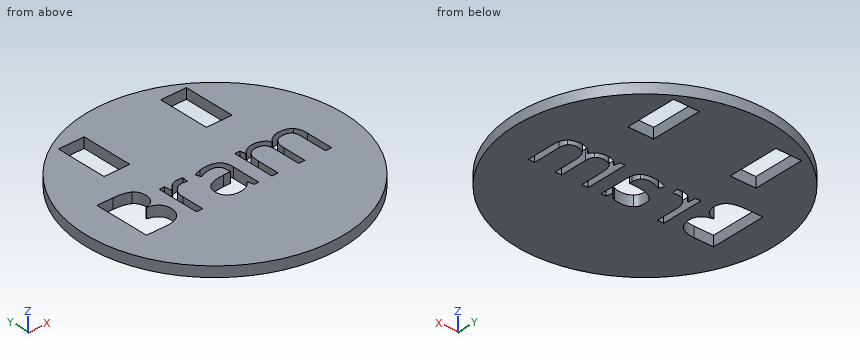
from build123d import *

# Parameters (mm, degrees)
F0_R     = 25
F0_W     = 5
F0_H     = 10
F1_DEPTH = 2


with BuildPart() as f1:
    # F0 (on Top) → F1 (new body)
    with BuildSketch(Plane.XY):
        Circle(F0_R)
        with BuildLine():
            Line((-18.475540486, -5.8509828523), (-18.475540486, 5.0045425299))
            Line((-18.475540486, 5.0045425299), (-15.4082427691, 5.0045425299))
            add(Edge.make_bspline(
                [(-15.4082427691, 5.0045425299), (-13.2485420529, 5.0045425299), (-12.2827352969, 4.3582954509)],
                knots=[0, 0, 0, 1, 1, 1], degree=2))
            add(Edge.make_bspline(
                [(-12.2827352969, 4.3582954509), (-11.316928541, 3.7120483719), (-11.316928541, 2.3173901536)],
                knots=[0, 0, 0, 1, 1, 1], degree=2))
            add(Edge.make_bspline(
                [(-11.316928541, 2.3173901536), (-11.316928541, 1.3503954435), (-11.8550717888, 0.7231556315)],
                knots=[0, 0, 0, 1, 1, 1], degree=2))
            add(Edge.make_bspline(
                [(-11.8550717888, 0.7231556315), (-12.3932150366, 0.0959158196), (-13.4267351813, -0.089405034)],
                knots=[0, 0, 0, 1, 1, 1], degree=2))
            Line((-13.4267351813, -0.089405034), (-13.4267351813, -0.1630581937))
            add(Edge.make_bspline(
                [(-13.4267351813, -0.1630581937), (-10.9534145591, -0.5859698851), (-10.9534145591, -2.76230196)],
                knots=[0, 0, 0, 1, 1, 1], degree=2))
            add(Edge.make_bspline(
                [(-10.9534145591, -2.76230196), (-10.9534145591, -4.2163578877), (-11.9370406278, -5.03367037)],
                knots=[0, 0, 0, 1, 1, 1], degree=2))
            add(Edge.make_bspline(
                [(-11.9370406278, -5.03367037), (-12.9206666966, -5.8509828523), (-14.6883425304, -5.8509828523)],
                knots=[0, 0, 0, 1, 1, 1], degree=2))
            Line((-14.6883425304, -5.8509828523), (-18.475540486, -5.8509828523))
        make_face(mode=Mode.SUBTRACT)
        with BuildLine():
            add(Edge.make_bspline(
                [(-6.4985863491, 2.0049582018), (-5.8594669952, 2.4361855726), (-5.0944244973, 2.4361855726)],
                knots=[0, 0, 0, 1, 1, 1], degree=2))
            add(Edge.make_bspline(
                [(-5.0944244973, 2.4361855726), (-4.5527173869, 2.4361855726), (-4.1226779704, 2.3459010542)],
                knots=[0, 0, 0, 1, 1, 1], degree=2))
            Line((-4.1226779704, 2.3459010542), (-4.2937433736, 1.203089124))
            add(Edge.make_bspline(
                [(-4.2937433736, 1.203089124), (-4.7974359499, 1.3147568178), (-5.1847090156, 1.3147568178)],
                knots=[0, 0, 0, 1, 1, 1], degree=2))
            add(Edge.make_bspline(
                [(-5.1847090156, 1.3147568178), (-6.1730869012, 1.3147568178), (-6.8739798729, 0.51288774)],
                knots=[0, 0, 0, 1, 1, 1], degree=2))
            add(Edge.make_bspline(
                [(-6.8739798729, 0.51288774), (-7.5748728446, -0.2889813378), (-7.5748728446, -1.4840632523)],
                knots=[0, 0, 0, 1, 1, 1], degree=2))
            Line((-7.5748728446, -1.4840632523), (-7.5748728446, -5.8509828523))
            Line((-7.5748728446, -5.8509828523), (-8.8079692931, -5.8509828523))
            Line((-8.8079692931, -5.8509828523), (-8.8079692931, 2.2865033447))
            Line((-8.8079692931, 2.2865033447), (-7.7910805071, 2.2865033447))
            Line((-7.7910805071, 2.2865033447), (-7.6485260043, 0.7801774326))
            Line((-7.6485260043, 0.7801774326), (-7.5891282949, 0.7801774326))
            add(Edge.make_bspline(
                [(-7.5891282949, 0.7801774326), (-7.1377057029, 1.5737308311), (-6.4985863491, 2.0049582018)],
                knots=[0, 0, 0, 1, 1, 1], degree=2))
        make_face(mode=Mode.SUBTRACT)
        with BuildLine():
            Line((3.3186670717, -5.8509828523), (2.4039423459, -5.8509828523))
            Line((2.4039423459, -5.8509828523), (2.1592237829, -4.6915395635))
            Line((2.1592237829, -4.6915395635), (2.0998260734, -4.6915395635))
            add(Edge.make_bspline(
                [(2.0998260734, -4.6915395635), (1.4915935284, -5.4565820614), (0.8869248461, -5.7286235708)],
                knots=[0, 0, 0, 1, 1, 1], degree=2))
            add(Edge.make_bspline(
                [(0.8869248461, -5.7286235708), (0.2822561637, -6.0006650801), (-0.625340837, -6.0006650801)],
                knots=[0, 0, 0, 1, 1, 1], degree=2))
            add(Edge.make_bspline(
                [(-0.625340837, -6.0006650801), (-1.8346782017, -6.0006650801), (-2.5213157231, -5.3758011765)],
                knots=[0, 0, 0, 1, 1, 1], degree=2))
            add(Edge.make_bspline(
                [(-2.5213157231, -5.3758011765), (-3.2079532446, -4.750937273), (-3.2079532446, -3.6009976177)],
                knots=[0, 0, 0, 1, 1, 1], degree=2))
            add(Edge.make_bspline(
                [(-3.2079532446, -3.6009976177), (-3.2079532446, -1.137180629), (0.7336787556, -1.01838521)],
                knots=[0, 0, 0, 1, 1, 1], degree=2))
            Line((0.7336787556, -1.01838521), (2.1140815237, -0.9732429509))
            Line((2.1140815237, -0.9732429509), (2.1140815237, -0.4671744662))
            add(Edge.make_bspline(
                [(2.1140815237, -0.4671744662), (2.1140815237, 0.4903166104), (1.7030493742, 0.9464910191)],
                knots=[0, 0, 0, 1, 1, 1], degree=2))
            add(Edge.make_bspline(
                [(1.7030493742, 0.9464910191), (1.2920172246, 1.4026654278), (0.384420224, 1.4026654278)],
                knots=[0, 0, 0, 1, 1, 1], degree=2))
            add(Edge.make_bspline(
                [(0.384420224, 1.4026654278), (-0.6324685621, 1.4026654278), (-1.9154590866, 0.7801774326)],
                knots=[0, 0, 0, 1, 1, 1], degree=2))
            Line((-1.9154590866, 0.7801774326), (-2.2956044272, 1.723413059))
            add(Edge.make_bspline(
                [(-2.2956044272, 1.723413059), (-1.6944996074, 2.0489125068), (-0.9781632312, 2.2342333604)],
                knots=[0, 0, 0, 1, 1, 1], degree=2))
            add(Edge.make_bspline(
                [(-0.9781632312, 2.2342333604), (-0.261826855, 2.4195542139), (0.4604492921, 2.4195542139)],
                knots=[0, 0, 0, 1, 1, 1], degree=2))
            add(Edge.make_bspline(
                [(0.4604492921, 2.4195542139), (1.9145052199, 2.4195542139), (2.6165861458, 1.7744950891)],
                knots=[0, 0, 0, 1, 1, 1], degree=2))
            add(Edge.make_bspline(
                [(2.6165861458, 1.7744950891), (3.3186670717, 1.1294359643), (3.3186670717, -0.2961090629)],
                knots=[0, 0, 0, 1, 1, 1], degree=2))
            Line((3.3186670717, -0.2961090629), (3.3186670717, -5.8509828523))
        make_face(mode=Mode.SUBTRACT)
        with BuildLine():
            Line((17.4600737416, -5.8509828523), (16.2293532014, -5.8509828523))
            Line((16.2293532014, -5.8509828523), (16.2293532014, -0.5574589846))
            add(Edge.make_bspline(
                [(16.2293532014, -0.5574589846), (16.2293532014, 0.4166634507), (15.8135692351, 0.9025367141)],
                knots=[0, 0, 0, 1, 1, 1], degree=2))
            add(Edge.make_bspline(
                [(15.8135692351, 0.9025367141), (15.3977852689, 1.3884099776), (14.5210750771, 1.3884099776)],
                knots=[0, 0, 0, 1, 1, 1], degree=2))
            add(Edge.make_bspline(
                [(14.5210750771, 1.3884099776), (13.3711354218, 1.3884099776), (12.8211126322, 0.7279074483)],
                knots=[0, 0, 0, 1, 1, 1], degree=2))
            add(Edge.make_bspline(
                [(12.8211126322, 0.7279074483), (12.2710898425, 0.067404919), (12.2710898425, -1.3058701239)],
                knots=[0, 0, 0, 1, 1, 1], degree=2))
            Line((12.2710898425, -1.3058701239), (12.2710898425, -5.8509828523))
            Line((12.2710898425, -5.8509828523), (11.037993394, -5.8509828523))
            Line((11.037993394, -5.8509828523), (11.037993394, -0.5574589846))
            add(Edge.make_bspline(
                [(11.037993394, -0.5574589846), (11.037993394, 0.4166634507), (10.6222094277, 0.9025367141)],
                knots=[0, 0, 0, 1, 1, 1], degree=2))
            add(Edge.make_bspline(
                [(10.6222094277, 0.9025367141), (10.2064254614, 1.3884099776), (9.3225875446, 1.3884099776)],
                knots=[0, 0, 0, 1, 1, 1], degree=2))
            add(Edge.make_bspline(
                [(9.3225875446, 1.3884099776), (8.1655201642, 1.3884099776), (7.6273769164, 0.694644731)],
                knots=[0, 0, 0, 1, 1, 1], degree=2))
            add(Edge.make_bspline(
                [(7.6273769164, 0.694644731), (7.0892336686, 0.0008794844), (7.0892336686, -1.5814754958)],
                knots=[0, 0, 0, 1, 1, 1], degree=2))
            Line((7.0892336686, -1.5814754958), (7.0892336686, -5.8509828523))
            Line((7.0892336686, -5.8509828523), (5.8561372201, -5.8509828523))
            Line((5.8561372201, -5.8509828523), (5.8561372201, 2.2865033447))
            Line((5.8561372201, 2.2865033447), (6.8587705559, 2.2865033447))
            Line((6.8587705559, 2.2865033447), (7.0583468597, 1.1722023151))
            Line((7.0583468597, 1.1722023151), (7.1177445692, 1.1722023151))
            add(Edge.make_bspline(
                [(7.1177445692, 1.1722023151), (7.4670031008, 1.7661794098), (8.1025585921, 2.1011824912)],
                knots=[0, 0, 0, 1, 1, 1], degree=2))
            add(Edge.make_bspline(
                [(8.1025585921, 2.1011824912), (8.7381140834, 2.4361855726), (9.5245397568, 2.4361855726)],
                knots=[0, 0, 0, 1, 1, 1], degree=2))
            add(Edge.make_bspline(
                [(9.5245397568, 2.4361855726), (11.4323941848, 2.4361855726), (12.0192435544, 1.0534068962)],
                knots=[0, 0, 0, 1, 1, 1], degree=2))
            Line((12.0192435544, 1.0534068962), (12.0786412638, 1.0534068962))
            add(Edge.make_bspline(
                [(12.0786412638, 1.0534068962), (12.4421552458, 1.69252625), (13.1323566298, 2.0643559113)],
                knots=[0, 0, 0, 1, 1, 1], degree=2))
            add(Edge.make_bspline(
                [(13.1323566298, 2.0643559113), (13.8225580138, 2.4361855726), (14.7063959307, 2.4361855726)],
                knots=[0, 0, 0, 1, 1, 1], degree=2))
            add(Edge.make_bspline(
                [(14.7063959307, 2.4361855726), (16.0867986987, 2.4361855726), (16.7734362201, 1.7269769215)],
                knots=[0, 0, 0, 1, 1, 1], degree=2))
            add(Edge.make_bspline(
                [(16.7734362201, 1.7269769215), (17.4600737416, 1.0177682705), (17.4600737416, -0.5432035343)],
                knots=[0, 0, 0, 1, 1, 1], degree=2))
            Line((17.4600737416, -0.5432035343), (17.4600737416, -5.8509828523))
        make_face(mode=Mode.SUBTRACT)
        with Locations((-10, 15.2066518739)):
            Rectangle(F0_W, F0_H, mode=Mode.SUBTRACT)
        with Locations((10, 15.3693027049)):
            Rectangle(F0_W, F0_H, mode=Mode.SUBTRACT)
    extrude(amount=F1_DEPTH)


solid = f1.part
CAD build for the part. Positions are in the model's coordinates, mm. Round coordinates to 2 decimals unless told otherwise and drop trailing zeros. Write each loop counter-clockwise with the first axis right and the second up, starting at its lowest first coordinate (ties: lowest second). Pieces come first, ordered by that corner, then holes. Notation, with made-up numbers: M -21,7 L -8,7 A21 cw -8,20 Z; hole C 43.5,-39 d6. An arc over 180 degrees is marked long. Put each result on its own line as item: value. Start each with the question number.
1) Saw through at D-D, the plane x = 22. Write the cut outline in (y, z).
2) Drill centre lines: probe 1 along Y at (x, z) = (0.5, 0.8) (1 decimal); probe 2 along Y at (x, z) = (-2, 0.55); probe 3 along X at (y, z) = (2.5, 0.6). Where is each one in solid material? Low to high. Write a range as [from, to].
3) Pin check, flat tips, straight feed: pin 1 Ø1 at (y, z) = (-3, 1.5) entering from +X; pin 2 Ø1 at (y, z) = (-3.5, 0.5) entering from -X; pin 3 Ø0.6 at (x, z) = (10, 1.5) entering from +Y. Stop position of each tip, or through.
4) Saw through at B-B, the plane z = 1.25. Count the separate pieces of the cut face and the enclosed holes in it, and give its area (3 significant figures).
5) Saw through at A-A, the plane y = 11. Write the cut outline in (x, z), and give its area (3 significant figures).
Resolved:
1. outline: M -11.87,0 L 11.87,0 L 11.87,2 L -11.87,2 Z
2. probe 1: [-25, -5.9], [-1, 1.4], [2.4, 25]
2. probe 2: [-24.92, -5.73], [-1.59, 0.99], [1.87, 24.92]
2. probe 3: [-24.87, -18.48], [-11.32, 24.87]
3. pin 1: x = 24.87
3. pin 2: x = -24.82
3. pin 3: y = 23.04
4. separate pieces: 1
4. enclosed holes: 6
4. area: 1,700 mm²
5. outline: M -22.45,0 L -12.5,0 L -12.5,2 L -22.45,2 Z; M -7.5,0 L 7.5,0 L 7.5,2 L -7.5,2 Z; M 12.5,0 L 22.45,0 L 22.45,2 L 12.5,2 Z
5. area: 69.8 mm²
